```python
from build123d import *
from build123d.topology import SkipClean

# Parameters (mm, degrees)
SKETCH1_R           = 93.345
SKETCH1_R_2         = 83.82
BOSS_EXTRUDE1_DEPTH = 15.875
SKETCH2_R           = 88.9
SKETCH2_R_2         = 83.82
BOSS_EXTRUDE2_DEPTH = 38.1
CUT_EXTRUDE1_DEPTH  = 38.1
CIRPATTERN1_COUNT   = 4
SKETCH4_R           = 88.9
SKETCH4_R_2         = 83.82
BOSS_EXTRUDE3_DEPTH = 15.875


with BuildPart() as part:
    # Sketch1 → Boss-Extrude1 (new, symmetric)
    with BuildSketch(Plane(origin=(0, 0, 0), x_dir=(1, 0, 0), z_dir=(0, 1, 0))):
        with Locations(Location((0, 0, 0), (0, 0, 270))):
            Circle(SKETCH1_R)
        with Locations(Location((0, 0, 0), (0, 0, 270))):
            Circle(SKETCH1_R_2, mode=Mode.SUBTRACT)
    extrude(amount=BOSS_EXTRUDE1_DEPTH, both=True)

    # Sketch2 → Boss-Extrude2 (add, symmetric)
    with BuildSketch(Plane(origin=(0, 0, 0), x_dir=(1, 0, 0), z_dir=(0, 1, 0))):
        with Locations(Location((0, 0, 0), (0, 0, 90))):
            Circle(SKETCH2_R)
        with Locations(Location((0, 0, 0), (0, 0, 270))):
            Circle(SKETCH2_R_2, mode=Mode.SUBTRACT)
    extrude(amount=BOSS_EXTRUDE2_DEPTH, both=True)

    # Sketch3 → Cut-Extrude1 (cut, symmetric)
    with BuildSketch(Plane(origin=(0, 0, 0), x_dir=(1, 0, 0), z_dir=(0, 1, 0))):
        with BuildLine():
            Line((0, 0), (-30.405590742, 83.538673988))
            ThreePointArc((-30.405590742, 83.538673988), (0, 88.9), (30.405590742, 83.538673988))
            Line((30.405590742, 83.538673988), (0, 0))
        make_face()
    cut_extrude1 = extrude(amount=CUT_EXTRUDE1_DEPTH, both=True, mode=Mode.SUBTRACT)

    # CirPattern1: Cut-Extrude1 ×4 about axis
    cirpattern1_axis = Axis((0, 38.1, 0), (0, -1, 0))
    for i in range(1, CIRPATTERN1_COUNT):
        add(cut_extrude1.rotate(cirpattern1_axis, i * 360 / CIRPATTERN1_COUNT), mode=Mode.SUBTRACT)

    # Sketch4 → Boss-Extrude3 (add, symmetric)
    with SkipClean():  # the faces are left unmerged after this step: merging them gives an invalid solid
        with BuildSketch(Plane(origin=(0, 0, 0), x_dir=(1, 0, 0), z_dir=(0, 1, 0))):
            Circle(SKETCH4_R)
            with Locations(Location((0, 0, 0), (0, 0, 110))):
                Circle(SKETCH4_R_2, mode=Mode.SUBTRACT)
        extrude(amount=BOSS_EXTRUDE3_DEPTH, both=True)


solid = part.part
```
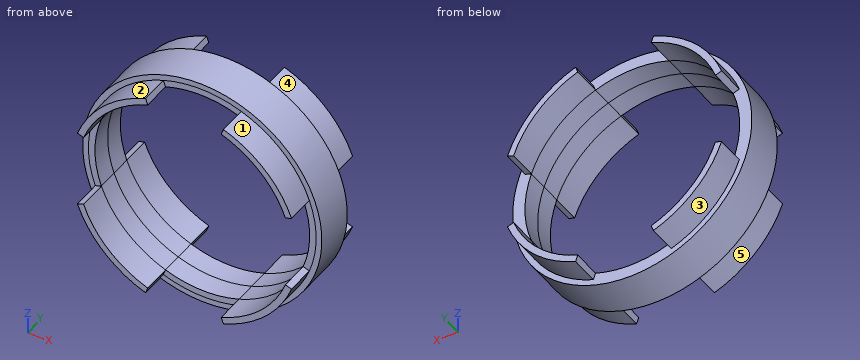
Could you check a few things on this model? Use its own coordinates, in mm. Face numbers are marked on the shaded views. A direction names the side the tool comes from. Coordinates: 2 decimals unless noted, no trailing zeros. Write each loop counter-clockwise with the first axis right and the second up, starting at its lowest first coordinate (ties: lowest second). Pieces come first, ordered by that corner, then holes. Notation, with made-up numbers: (9, 14) -> (42, 14) arc R24 ccw to (42, 38) -> close; hole circle Ø2 at (73.5, 63.5). An arc over 180 degrees is marked (long way). One line per question, with ' | ' between items. Start each with the question number.
1. If we section it at C-C (x = 0): Please give me the cut outline in (y, z) (3 decimals).
2. Will these pins go through, and if not, where does the flat tip stop? P1, Ø8, axis at x = -11, z = 81.5, coming from the -Y side (3 decimals); P2, Ø3, axis at x = 67.5, y = 0, coming from the -Z side.
3. If we section it at A-A (z = 0): Please give me the cut outline in (x, y) (3 decimals), and give its area (3 significant figures).
4. If we section it at D-D (z = -46): Please give me the cut outline in (x, y) (3 decimals), and give its area (3 significant figures).
5. If we section it at B-B (y = -30): Please give me the cut outline in (x, z), and give its area (3 significant figures).
6. For the marked faces 1, 2, 3, 4 and 5, which set-ups out of +Z, -Z, +X, -X, +Y, -Y let a thin tool reach every point of the face, with its end or its side?
7. Please list where these lines run through material, in increasing order: line 1 along X through (y, z) = (-32, 58); line 2 along X through (y, z) = (15.5, 57); line 3 along Z through (x, y) = (-15.5, -3).
Return value:
1) outline: (-15.875, -93.345) -> (15.875, -93.345) -> (15.875, -83.82) -> (-15.875, -83.82) -> close; (-15.875, 83.82) -> (15.875, 83.82) -> (15.875, 93.345) -> (-15.875, 93.345) -> close
2) P1: stops at y = -15.875 | P2: stops at z = -66.01
3) outline: (-93.345, -15.875) -> (-83.82, -15.875) -> (-83.82, 15.875) -> (-93.345, 15.875) -> close; (83.82, -15.875) -> (93.345, -15.875) -> (93.345, 15.875) -> (83.82, 15.875) -> close | area: 605 mm²
4) outline: (-81.224, -15.875) -> (-76.074, -15.875) -> (-76.074, -38.1) -> (-70.07, -38.1) -> (-70.07, 38.1) -> (-76.074, 38.1) -> (-76.074, 15.875) -> (-81.224, 15.875) -> close; (70.07, -38.1) -> (76.074, -38.1) -> (76.074, -15.875) -> (81.224, -15.875) -> (81.224, 15.875) -> (76.074, 15.875) -> (76.074, 38.1) -> (70.07, 38.1) -> close | area: 1,240 mm²
5) outline: (-83.54, -30.41) arc R88.9 ccw to (-30.41, -83.54) -> (-28.67, -78.77) arc R83.82 cw to (-78.77, -28.67) -> close; (-83.54, 30.41) -> (-78.77, 28.67) arc R83.82 cw to (-28.67, 78.77) -> (-30.41, 83.54) arc R88.9 ccw to start; (28.67, -78.77) -> (30.41, -83.54) arc R88.9 ccw to (83.54, -30.41) -> (78.77, -28.67) arc R83.82 cw to start; (28.67, 78.77) arc R83.82 cw to (78.77, 28.67) -> (83.54, 30.41) arc R88.9 ccw to (30.41, 83.54) -> close | area: 1,530 mm²
6) face 1: +Z, +X, -Y | face 2: +Z, -X, -Y | face 3: -Z, -X, +Y | face 4: +Z, +X, +Y | face 5: -Z, -X, -Y
7) line 1: x = -67.37 to -60.51, 60.51 to 67.37 | line 2: x = -73.92 to -61.46, 61.46 to 73.92 | line 3: z = -92.05 to -82.37, 82.37 to 92.05
